For this review, take the finished solid that the model builds, in its own axes (mm). A direction names the side the tool comes from. Give positions to 0.01 mm unless a question says otherwise; leave off trailing zeros. Loops run counter-clockwise (first coordinate to the right, second up) from the corner with the lowest first, then second, coordinate; pieces in that order, holes last. Notation, with made-up numbers: (37.5, 6.5) - (93.5, 6.5) arc R3 ccw to (93.5, 10.5) - close; hole circle Ø2 at (80, 34.25). An arc over 180 degrees is marked (long way). Put each result on its own line as item: value.
from build123d import *

# Parameters (mm, degrees)
CROQUIS1_R              = 84
CROQUIS1_R_2            = 82
SALIENTE_EXTRUIR1_DEPTH = 10
CROQUIS2_R              = 84
SALIENTE_EXTRUIR2_DEPTH = 4
CROQUIS3_R              = 1.5
SALIENTE_EXTRUIR3_DEPTH = 10
MATRIZC1_COUNT          = 4
CROQUIS15_R             = 83
CROQUIS15_R_2           = 82
CORTAR_EXTRUIR1_DEPTH   = 5
CROQUIS16_R             = 18.5
CORTAR_EXTRUIR2_DEPTH   = 13


with BuildPart() as part:
    # Croquis1 → Saliente-Extruir1 (new body)
    with BuildSketch(Plane(origin=(0, 0, 0), x_dir=(1, 0, 0), z_dir=(0, 1, 0))):
        with Locations(Location((0, 0, 0), (0, 0, 270))):
            Circle(CROQUIS1_R)
        with Locations(Location((0, 0, 0), (0, 0, 270))):
            Circle(CROQUIS1_R_2, mode=Mode.SUBTRACT)
    extrude(amount=SALIENTE_EXTRUIR1_DEPTH)

    # Croquis2 → Saliente-Extruir2 (add)
    with BuildSketch(Plane(origin=(0, 10, 0), x_dir=(1, 0, 0), z_dir=(0, 1, 0))):
        with Locations(Location((0, 0, 0), (0, 0, 270))):
            Circle(CROQUIS2_R)
    extrude(amount=SALIENTE_EXTRUIR2_DEPTH)

    # Croquis3 → Saliente-Extruir3 (add)
    with BuildSketch(Plane.XZ.offset(-10)):
        with Locations(Location((-20, 40, 0), (0, 0, 90))):
            Circle(CROQUIS3_R)
    saliente_extruir3 = extrude(amount=SALIENTE_EXTRUIR3_DEPTH)

    # MatrizC1: Saliente-Extruir3 ×4 about axis
    matrizc1_axis = Axis((0, 0, 0), (0, 1, 0))
    for i in range(1, MATRIZC1_COUNT):
        add(saliente_extruir3.rotate(matrizc1_axis, i * 360 / MATRIZC1_COUNT))

    # Croquis15 → Cortar-Extruir1 (cut)
    with BuildSketch(Plane.XZ):
        with Locations(Location((0, 0, 0), (0, 0, 270))):
            Circle(CROQUIS15_R)
        with Locations(Location((0, 0, 0), (0, 0, 270))):
            Circle(CROQUIS15_R_2, mode=Mode.SUBTRACT)
    extrude(amount=-CORTAR_EXTRUIR1_DEPTH, mode=Mode.SUBTRACT)

    # Croquis16 → Cortar-Extruir2 (cut)
    with BuildSketch(Plane.XZ.offset(-10)):
        with Locations(Location((0, 0, 0), (0, 0, 270))):
            Circle(CROQUIS16_R)
    extrude(amount=-CORTAR_EXTRUIR2_DEPTH, mode=Mode.SUBTRACT)


solid = part.part
1) Take a section at B-B on x = 0. State the section outline as (y, z) points.
Geometry check:
outline: (0, -84) - (14, -84) - (14, -18.5) - (10, -18.5) - (10, -82) - (5, -82) - (5, -83) - (0, -83) - close; (0, 83) - (5, 83) - (5, 82) - (10, 82) - (10, 18.5) - (14, 18.5) - (14, 84) - (0, 84) - close
2) Insertion check: pin 1 Ø5 at (y, z) = (6.5, 64) entering from -X; pin 2 Ø1.5 at (x, z) = (-32.5, 52.5) entering from -Y; pin 3 Ø8 at (y, z) = (3.5, 22.5) entering from -X; pin 4 Ø22 at (x, z) = (0, 0) entering from +Y. Each pin has a flat end and moves straight along its axis. Give the tip position at first contact, or say it passes through.
Geometry check:
pin 1: stops at x = -57.22
pin 2: stops at y = 10
pin 3: stops at x = -81.94
pin 4: passes through
3) Take a section at A-A on z = 0. State the section outline as (x, y) points, and give its area (3 significant figures).
Geometry check:
outline: (-84, 0) - (-83, 0) - (-83, 5) - (-82, 5) - (-82, 10) - (-18.5, 10) - (-18.5, 14) - (-84, 14) - close; (18.5, 10) - (82, 10) - (82, 5) - (83, 5) - (83, 0) - (84, 0) - (84, 14) - (18.5, 14) - close
area: 554 mm²
4) Draft analysis for pull direction X (two halves, no side actions). For faces 3 (the face through (24.931, 2.465, -79.167)), 4 (the face through (25.23, 6.9, 80.12)), 5 (the face through (81, 0, -19)), state which applies: pulls with the +X half, pulls with the -X half, needs draft (parallel to the pull), parting line crosses it, or undercut.
Geometry check:
face 3: undercut
face 4: parting line crosses it
face 5: needs draft
5) Wall thickness on line 1 (X direction, y = 12.25, z = 0); line 2 (X direction, y = 8.25, z = -0.5); line 3 (Y direction, x = 62, z = -44.5): over which ranges is each line inside the solid? List them lowest first.
Geometry check:
line 1: x = -84 to -18.5, 18.5 to 84
line 2: x = -84 to -82, 82 to 84
line 3: y = 10 to 14
6) Take a section at C-C on x = 52. State the section outline as (y, z) points, and give its area (3 significant figures).
Geometry check:
outline: (0, -65.97) - (14, -65.97) - (14, 65.97) - (0, 65.97) - (0, 64.69) - (5, 64.69) - (5, 63.4) - (10, 63.4) - (10, -63.4) - (5, -63.4) - (5, -64.69) - (0, -64.69) - close
area: 566 mm²
7) For faces 1 (the face through (20, 14, -1)), 2 (the face through (19, 5, 80)), list the 3-axis set-ups (+Z, -Z, +X, -X, +Y, -Y) from which the entire face can be reached by the end or side of a thin tool; tool diameter is ignored.
Geometry check:
face 1: +Z, -Z, +X, -X, +Y
face 2: -Y
8) Take a section at D-D on z = 70. State the section outline as (x, y) points, and give its area (3 significant figures).
Geometry check:
outline: (-46.43, 0) - (-44.6, 0) - (-44.6, 5) - (-42.71, 5) - (-42.71, 10) - (42.71, 10) - (42.71, 5) - (44.6, 5) - (44.6, 0) - (46.43, 0) - (46.43, 14) - (-46.43, 14) - close
area: 427 mm²
